Autodesk Inventor part; units mm, degrees
ref_plane "YZ Plane" through (0, 0, 0) normal (1, 0, 0) x (0, 1, 0)
ref_plane "XZ Plane" through (0, 0, 0) normal (0, 1, 0) x (-1, 0, 0)
ref_plane "XY Plane" through (0, 0, 0) normal (0, 0, 1) x (1, 0, 0)
sketch "Sketch3" plane through (0, 0, 0) normal (0, 1, 0) x (-1, 0, 0)
  line L0 (-74.2, 0) -> (-74.2, -26)
  line L1 (0, -26) -> (0, 0)
  line L2 (0, 0) -> (-24, 0)
  line L3 (-24, 0) -> (-24, 14.5)
  line L4 (-24, 14.5) -> (-50.2, 14.5)
  line L5 (-50.2, 14.5) -> (-50.2, 0)
  line L6 (-50.2, -26) -> (-50.2, -40.5)
  line L7 (-50.2, -40.5) -> (-24, -40.5)
  line L8 (-24, -40.5) -> (-24, -26)
  line L9 (0, -13) -> (-13.4, -13)
  line L10 (-74.2, -13) -> (-60.8, -13)
  line L11 (0, 0) -> (-24, 0)
  line L12 (-50.2, 0) -> (-74.2, 0)
  line L13 (-74.2, -26) -> (-50.2, -26)
  line L14 (-24, -26) -> (0, -26)
  circle A0 centre (-13.4, -13) radius 1.2
  circle A1 centre (-60.8, -13) radius 1.2
  dimension "d2" = 74.2
  dimension "d3" = 26
  dimension "d4" = 24
  dimension "d5" = 14.5
  dimension "d6" = 26.2
  dimension "d7" = 14.5
  dimension "d8" = 26.2
  dimension "d9" = 13.4
  dimension "d10" = 13.4
  dimension "d11" = 2.4
  dimension "d12" = 2.4
extrude "Extrusion1" add sketch "Sketch3" along normal blind 2.5
sketch "Sketch4" plane through (50.2, 0, 14.5) normal (1, 0, 0) x (0, 0, -1)
  point P0 (14.5, 0)
sketch "Sketch5" plane through (0, 2.5, 0) normal (0, 1, 0) x (1, 0, 0)
  line L0 (24, -14.5) -> (50.2, -14.5)
  line L1 (24, -14.5) -> (21.5, -14.5)
  line L2 (21.5, -14.5) -> (21.5, 0)
  line L3 (21.5, 0) -> (24, 0)
  line L4 (24, 0) -> (24, -14.5)
  point P0 (0, 0)
  dimension "d15" = 2.5
extrude "Extrusion2" add sketch "Sketch5" against normal blind 6.8
sketch "Sketch6" plane through (0, 2.5, 0) normal (0, 1, 0) x (1, 0, 0)
  line L0 (50.2, -14.5) -> (50.2, 0)
  line L1 (50.2, -14.5) -> (52.7, -14.5)
  line L2 (52.7, -14.5) -> (52.7, 0)
  line L3 (50.2, 0) -> (74.2, 0)
  line L4 (50.2, 0) -> (50.2, -14.5)
  point P0 (0, 0)
  dimension "d18" = 2.5
extrude "Extrusion3" add sketch "Sketch6" against normal blind 6.8
sketch "Sketch7" plane through (0, 2.5, 0) normal (0, 1, 0) x (1, 0, 0)
  line L0 (24, 40.5) -> (24, 26)
  line L1 (24, 40.5) -> (21.5, 40.5)
  line L2 (21.5, 40.5) -> (21.5, 26)
  line L3 (21.5, 26) -> (24, 26)
  line L4 (24, 26) -> (24, 40.5)
  point P0 (0, 0)
  dimension "d21" = 2.5
extrude "Extrusion4" add sketch "Sketch7" against normal blind 6.8
sketch "Sketch8" plane through (0, 2.5, 0) normal (0, 1, 0) x (1, 0, 0)
  line L0 (50.2, 26) -> (50.2, 40.5)
  line L1 (50.2, 40.5) -> (52.7, 40.5)
  line L2 (52.7, 40.5) -> (52.7, 26)
  line L3 (52.7, 26) -> (50.2, 26)
  line L4 (50.2, 26) -> (50.2, 40.5)
  point P0 (0, 0)
  dimension "d24" = 2.5
extrude "Extrusion5" add sketch "Sketch8" against normal blind 6.8
sketch "Sketch9" plane through (24, 0, -26) normal (1, 0, 0) x (0, 0, -1)
  line L0 (14.5, 0) -> (14.5, -4.3)
  line L1 (14.5, -4.3) -> (14.5, -1.8)
  line L2 (14.5, -1.8) -> (0, -1.8)
  line L3 (0, -1.8) -> (0, -4.3)
  line L4 (0, -4.3) -> (14.5, -4.3)
  point P0 (-26, 0)
  dimension "d27" = 2.5
extrude "Extrusion6" add sketch "Sketch9" along normal blind 5.8
sketch "Sketch10" plane through (50.2, 0, -40.5) normal (-1, 0, 0) x (0, 0, 1)
  line L0 (0, 0) -> (0, -4.3)
  line L1 (0, -4.3) -> (0, -1.8)
  line L2 (0, -1.8) -> (14.5, -1.8)
  line L3 (14.5, 0) -> (14.5, -4.3)
  line L4 (14.5, -1.8) -> (14.5, -4.3)
  line L5 (14.5, -4.3) -> (0, -4.3)
  point P0 (40.5, 0)
  dimension "d30" = 2.5
extrude "Extrusion7" add sketch "Sketch10" along normal blind 5.8
sketch "Sketch11" plane through (50.2, 0, 0) normal (-1, 0, 0) x (0, 0, 1)
  line L0 (14.5, -4.3) -> (0, -4.3)
  line L1 (0, -4.3) -> (0, -1.8)
  line L2 (0, 0) -> (0, -4.3)
  arc A0 (-2.0781, -1.1028) -> (0, -1.8) centre (0, 1.6455) ccw
  line L3 (0, -1.8) -> (14.5, -1.8)
  line L4 (14.5, -1.8) -> (14.5, -4.3)
  line L5 (0, 0) -> (0, -4.3)
  line L6 (14.5, 2.5) -> (14.5, -4.3)
  line L7 (0, -4.3) -> (14.5, -4.3)
  dimension "d33" = 2.5
extrude "Extrusion8" add sketch "Sketch11" along normal blind 5.8
sketch "Sketch12" plane through (24, 0, 14.5) normal (1, 0, 0) x (0, 0, -1)
  line L0 (0, 0) -> (0, -4.3)
  line L1 (0, -4.3) -> (0, -1.8)
  line L2 (0, -1.8) -> (14.5, -1.8)
  line L3 (14.5, -4.3) -> (0, -4.3)
  line L4 (14.5, -1.8) -> (14.5, -4.3)
  line L5 (14.5, -4.3) -> (0, -4.3)
  point P0 (14.5, 0)
  dimension "d36" = 2.5
extrude "Extrusion9" add sketch "Sketch12" along normal blind 5.8
properties part number "cam_holder"
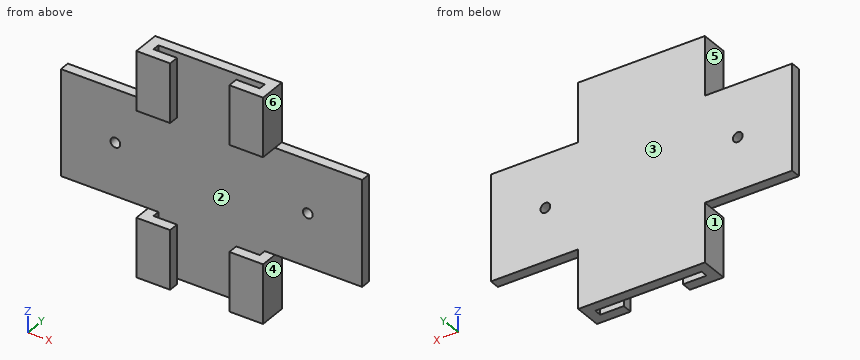
For this review, take the finished solid that the model builds, in its own axes (mm). Face numbers are marked on the shaded views. A direction names the side the tool comes from. Coordinates: 2 decimals unless noted, no trailing zeros. Write each loop counter-clockwise with the first axis right and the second up, starting at its lowest first coordinate (ties: lowest second). Pieces come first, ordered by that corner, then holes.
(1) Add section A-A on z = -13. Give the boundary of the cut face in (x, y).
(2) The part is to be moulded in two halves that separate along X. For the marked faces 1, 2 and 3, say which applies: +X half, -X half, draft (parallel to the pull), parting line (faces both ways), or undercut.
(3) Wall thickness on probe 1 along Z at (x, y) = (60.8, 1.7); probe 2 along X at (y, z) = (-2, -37); probe 3 along Y at (x, z) = (46, 6): over which ranges is each line inside the solid? List them lowest first.
(4) Add section D-D on z = -24. Give the boundary of the cut face in (x, y).
(5) Add section C-C on x = 51. Give the boundary of the cut face in (y, z), then the cut area to 3 significant figures.
(6) Add section B-B on x = 13.4. Give the boundary of the cut face in (y, z), then the cut area to 3 significant figures.
(7) Tool access review of the marked faces 4, 5 and 6: name each direction out of +Z, -Z, +X, -X, +Y, -Y from which nothing blocks a thin tool from reaching the whole face with its end or side.
(8) For pin 1 Ø1.2 at (y, z) = (-3.5, -33.5) entering from +X; pin 2 Ø2 at (x, y) = (15, -0.5) entering from -Z; pin 3 Ø1.2 at (y, z) = (-3, 5) entering from -X; pin 4 Ø2 at (y, z) = (-0.5, -5.5) entering from +X, all flat-tipped, find the tip position at first contact; note any pin that passes through.
Answer sheet:
1. outline: (0, 0) - (12.2, 0) - (12.2, 2.5) - (0, 2.5) - close; (14.6, 0) - (59.6, 0) - (59.6, 2.5) - (14.6, 2.5) - close; (62, 0) - (74.2, 0) - (74.2, 2.5) - (62, 2.5) - close
2. face 1: -X half
2. face 2: undercut
2. face 3: draft
3. probe 1: z = -26 to -14.2, -11.8 to 0
3. probe 2: x = 21.5 to 29.8, 44.4 to 52.7
3. probe 3: y = -4.3 to -1.8, 0 to 2.5
4. outline: (0, 0) - (74.2, 0) - (74.2, 2.5) - (0, 2.5) - close
5. outline: (-4.3, -40.5) - (2.5, -40.5) - (2.5, 14.5) - (-4.3, 14.5) - (-4.3, 0) - (0, 0) - (0, -26) - (-4.3, -26) - close
5. area: 262 mm2
6. outline: (0, -26) - (2.5, -26) - (2.5, -14.2) - (0, -14.2) - close; (0, -11.8) - (2.5, -11.8) - (2.5, 0) - (0, 0) - close
6. area: 59.0 mm2
7. face 4: -Z, +X, +Y, -Y
7. face 5: +Z, -X, +Y, -Y
7. face 6: +Z, +X, +Y, -Y
8. pin 1: stops at x = 52.7
8. pin 2: stops at z = -26
8. pin 3: stops at x = 21.5
8. pin 4: stops at x = 74.2
